Work out the finished part from the listing and answer in its coordinate system (mm). Face numbers are marked on the shaded views. A direction names the side the tool comes from. Round coordinates to 2 decimals unless told otherwise and drop trailing zeros. Loops run counter-clockwise (first coordinate to the right, second up) from the corner with the lowest first, then second, coordinate; pieces in that order, holes last. Notation, with made-up numbers: (-14.5, -25) -> (17.5, -25) arc R9 ccw to (17.5, -17) -> close; hole circle Ø7 at (-2, -5). An arc over 180 degrees is marked (long way). Use one line per item in the form item = value.
```python
from build123d import *

# Parameters (mm, degrees)
CYLINDER_R             = 10
CYLINDER_DEPTH         = 10
CYLINDER001_R          = 2
CYLINDER001_DEPTH      = 30
CYLINDER001_ROLL_ANGLE = -90
BOX002_W               = 10
BOX002_H               = 2.5
BOX002_DEPTH           = 10
BOX003_W               = 10
BOX003_H               = 2.5
BOX003_DEPTH           = 10
PAD_DEPTH              = 2.5
BOX004_W               = 15
BOX004_H               = 10
BOX004_DEPTH           = 10
BOX001_W               = 15
BOX001_H               = 5
BOX001_DEPTH           = 10
BOX_W                  = 40
BOX_H                  = 30
BOX_DEPTH              = 10


with BuildPart() as cylinder:
    # Cylinder → Cylinder (new body)
    with BuildSketch(Plane.XY.offset(-5)):
        Circle(CYLINDER_R)
    extrude(amount=CYLINDER_DEPTH)


with BuildPart() as cylinder001:
    # Cylinder001 → Cylinder001 (new body)
    with BuildSketch(Plane.XY):
        Circle(CYLINDER001_R)
    extrude(amount=CYLINDER001_DEPTH)


with BuildPart() as cylinder001_1:
    # Cylinder001 roll: moved
    add(cylinder001.part.rotate(Axis((0, 0, 0), (1, 0, 0)), CYLINDER001_ROLL_ANGLE))


with BuildPart() as cylinder001_2:
    # Cylinder001 placement: moved
    add(cylinder001_1.part.moved(Location((-15, -15, 0))))


with BuildPart() as cube002:
    # Box002 → Box002 (new body)
    with BuildSketch(Plane(origin=(-20, 12.5, -5), x_dir=(1, 0, 0), z_dir=(0, 0, 1))):
        with Locations((5, 1.25)):
            Rectangle(BOX002_W, BOX002_H)
    extrude(amount=BOX002_DEPTH)


with BuildPart() as cube003:
    # Box003 → Box003 (new body)
    with BuildSketch(Plane(origin=(-20, -15, -5), x_dir=(1, 0, 0), z_dir=(0, 0, 1))):
        with Locations((5, 1.25)):
            Rectangle(BOX003_W, BOX003_H)
    extrude(amount=BOX003_DEPTH)


with BuildPart() as body:
    # Sketch → Pad (new body)
    with BuildSketch(Plane.XZ):
        Polygon((0, -4.041452), (3.5, -2.020726), (3.5, 2.020726), (0, 4.041452), (-3.5, 2.020726), (-3.5, -2.020726), align=None)
    extrude(amount=-PAD_DEPTH)


with BuildPart() as body_1:
    # Body placement: moved
    add(body.part.moved(Location((-15, -12.5, 0))))


with BuildPart() as cube004:
    # Box004 → Box004 (new body)
    with BuildSketch(Plane(origin=(0, -5, -5), x_dir=(1, 0, 0), z_dir=(0, 0, 1))):
        with Locations((7.5, 5)):
            Rectangle(BOX004_W, BOX004_H)
    extrude(amount=BOX004_DEPTH)


with BuildPart() as negative_fusion:
    # Box001 → Box001 (new body)
    with BuildSketch(Plane(origin=(-20, -2.5, -5), x_dir=(1, 0, 0), z_dir=(0, 0, 1))):
        with Locations((7.5, 2.5)):
            Rectangle(BOX001_W, BOX001_H)
    extrude(amount=BOX001_DEPTH)

    # Fusion: union Cylinder, Cylinder001, Cube002, Cube003, Body, Cube004
    add(cylinder.part)
    add(cylinder001_2.part)
    add(cube002.part)
    add(cube003.part)
    add(body_1.part)
    add(cube004.part)


with BuildPart() as cut:
    # Box → Box (new body)
    with BuildSketch(Plane(origin=(-20, -15, -5), x_dir=(1, 0, 0), z_dir=(0, 0, 1))):
        with Locations((20, 15)):
            Rectangle(BOX_W, BOX_H)
    extrude(amount=BOX_DEPTH)

    # Cut: cut Negative Fusion
    add(negative_fusion.part, mode=Mode.SUBTRACT)


solid = cut.part
```
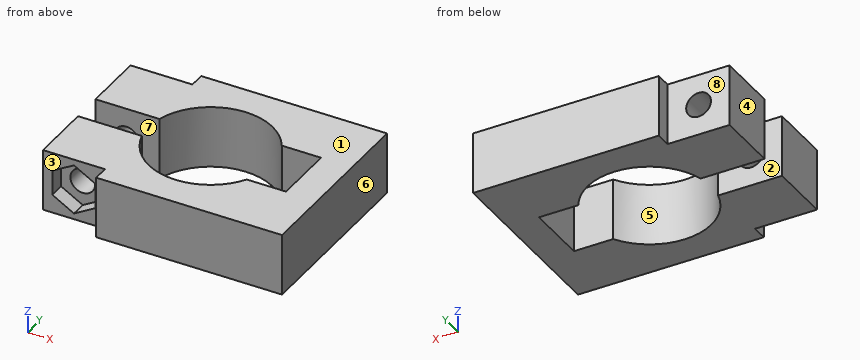
(1) For the marked faces 4, 5, 6, 7 and 8, determine the directions among +Z, -Z, +X, -X, +Y, -Y from which every point of the face is accessible in a straight line to the end or side of a thin tool.
Completed:
face_4 = +Z, -Z, -X, +Y, -Y
face_5 = +Z, -Z
face_6 = +Z, -Z, +X, +Y, -Y
face_7 = +Z, -Z, -X
face_8 = +Z, -Z, -X, +Y
(2) Given P1, Ø3, axis at x = -16.5, z = 0.5, coming from the +Y side; P2, Ø3.5, axis at x = -15, z = 0, coming from the +Y side; P3, Ø5, axis at x = -13, z = 0.5, coming from the -Y side; P4, Ø5, axis at x = -15.5, z = 0.5, coming from the -Y side, each flat-ended and moving along its own axis, determine where each tip first touches the part or whether it passes through.
Completed:
P1 = 12.5
P2 = through
P3 = -12.5
P4 = -10
(3) Find section A-A, the plane x = 13.5. Write down the section's boundary in (y, z), then the cut area to 3 significant figures.
Completed:
outline = (-15, -5) -> (-5, -5) -> (-5, 5) -> (-15, 5) -> close; (5, -5) -> (15, -5) -> (15, 5) -> (5, 5) -> close
area = 200 mm2
(4) For a pull along Y with two mould halves and no side action, classify the marked faces 1, 2 and 3 as +Y half, -Y half, draft (parallel to the pull), parting line (faces both ways), or undercut.
Completed:
face_1 = draft
face_2 = undercut
face_3 = -Y half
(5) Consider L1, parallel to Y at x = -16, z = -2.5; L2, parallel to Z at x = -15, y = -4.5; L3, parallel to Y at x = 6, z = -1.25. Determine where each line is inside the solid, lowest interval first.
Completed:
L1 = -10 to -2.5, 2.5 to 12.5
L2 = -5 to -2, 2 to 5
L3 = -15 to -8, 8 to 15
(6) Find section B-B, the plane z = 0. Write down the section's boundary in (x, y), then the cut area to 3 significant figures.
Completed:
outline = (-20, -12.5) -> (-18.5, -12.5) -> (-18.5, -10) -> (-17, -10) -> (-17, -2.5) -> (-20, -2.5) -> close; (-20, 2.5) -> (-17, 2.5) -> (-17, 12.5) -> (-20, 12.5) -> close; (-13, -10) -> (-11.5, -10) -> (-11.5, -12.5) -> (-10, -12.5) -> (-10, -15) -> (20, -15) -> (20, 15) -> (-10, 15) -> (-10, 12.5) -> (-13, 12.5) -> (-13, 2.5) -> (-9.68, 2.5) arc R10 cw to (8.66, 5) -> (15, 5) -> (15, -5) -> (8.66, -5) arc R10 cw to (-9.68, -2.5) -> (-13, -2.5) -> close
area = 643 mm2
(7) Find section C-C, the plane y = -7.25. Write down the section's boundary in (x, z).
Completed:
outline = (-20, -5) -> (-6.89, -5) -> (-6.89, 5) -> (-20, 5) -> close; (6.89, -5) -> (20, -5) -> (20, 5) -> (6.89, 5) -> close; hole circle Ø4 at (-15, 0)
(8) Find section D-D, the plane x = 1. Write down the section's boundary in (y, z).
Completed:
outline = (-15, -5) -> (-9.95, -5) -> (-9.95, 5) -> (-15, 5) -> close; (9.95, -5) -> (15, -5) -> (15, 5) -> (9.95, 5) -> close
